from build123d import *

# Parameters (mm, degrees)
SKETCH1_R           = 5
BOSS_EXTRUDE1_DEPTH = 18
SKETCH2_R           = 2.27
CUT_EXTRUDE1_DEPTH  = 5.68
CUT_EXTRUDE1_TAPER  = 3.074
SKETCH7_R           = 1
CUT_EXTRUDE2_DEPTH  = 19
SKETCH9_R           = 2.27
CUT_EXTRUDE3_DEPTH  = 5.68
CUT_EXTRUDE3_TAPER  = 3.074


with BuildPart() as part:
    # Sketch1 → Boss-Extrude1 (new body)
    with BuildSketch(Plane.XY):
        Circle(SKETCH1_R)
    extrude(amount=BOSS_EXTRUDE1_DEPTH)

    # Sketch2 → Cut-Extrude1 (cut)
    with BuildSketch(Plane.XY):
        Circle(SKETCH2_R)
    extrude(amount=CUT_EXTRUDE1_DEPTH, taper=CUT_EXTRUDE1_TAPER, mode=Mode.SUBTRACT)

    # Sketch7 → Cut-Extrude2 (cut, through all)
    with BuildSketch(Plane.XY):
        Circle(SKETCH7_R)
    extrude(amount=CUT_EXTRUDE2_DEPTH, mode=Mode.SUBTRACT)

    # Sketch9 → Cut-Extrude3 (cut)
    with BuildSketch(Plane.XY.offset(18)):
        Circle(SKETCH9_R)
    extrude(amount=-CUT_EXTRUDE3_DEPTH, taper=CUT_EXTRUDE3_TAPER, mode=Mode.SUBTRACT)


solid = part.part
Here's how the part is built. I have some questions about the finished solid (model axes, mm). A direction names the side the tool comes from. Round coordinates to 2 decimals unless told otherwise and drop trailing zeros. Write each loop counter-clockwise with the first axis right and the second up, starting at its lowest first coordinate (ties: lowest second). Pieces come first, ordered by that corner, then holes.
1. Suppose I cut it at C-C (z = 16.25). List the corners of the cut face in (x, y) for me, and give its area (3 significant figures).
2. Suppose I cut it at D-D (z = 10.5). List the corners of the cut face in (x, y) for me.
3. I need wall thicknesses on L1, parallel to Y at x = 0, z = 9.5; L2, parallel to Y at x = -0.5, z = 1.75; L3, parallel to X at y = 1.5, z = 5. Which ranges of each line are inside material? Lowest first, please.
4. Will these pins go through, and if not, where does the flat tip stop? pin 1 Ø1 at (y, z) = (-3, 14.5) entering from -X; pin 2 Ø5 at (y, z) = (-1.5, 10) entering from -X; pin 3 Ø1 at (x, z) = (2.5, 5.5) entering from +Y; pin 4 Ø1.2 at (x, y) = (1, 0) entering from +Z.
5. Suppose I cut it at A-A (x = 0). List the corners of the cut face in (y, z) for me, and give its area (3 significant figures).
6. For faces 1 (the flat face through (1, -1, 12.32)), 2 (the conical face through (2.018, 0.635, 2.88)), which set-ups out of +Z, -Z, +X, -X, +Y, -Y let a thin tool reach every point of the face, with its end or its side?
7. If we mould it in two halves opening along Y, with no side actions, what happens to faces 3 (the flat face through (2.2, 1.2, 0)), 4 (the cylindrical face through (-1.08, -4.88, 8.87)), 5 (the flat face through (1, -1, 5.68))? For each: released by +Y, released by -Y, zero draft, split by the parting line, or undercut.
8. Suppose I cut it at B-B (y = 3). List the corners of the cut face in (x, z) for me, and give its area (3 significant figures).
Answer sheet:
1. outline: circle Ø10 at (0, 0); hole circle Ø4.35 at (0, 0)
1. area: 63.7 mm2
2. outline: circle Ø10 at (0, 0); hole circle Ø2 at (0, 0)
3. L1: y = -5 to -1, 1 to 5
3. L2: y = -4.97 to -2.12, 2.12 to 4.97
3. L3: x = -4.77 to -1.33, 1.33 to 4.77
4. pin 1: stops at x = -4.33
4. pin 2: stops at x = -5
4. pin 3: stops at y = 4.58
4. pin 4: stops at z = 12.32
5. outline: (-5, 0) - (-2.27, 0) - (-1.96, 5.68) - (-1, 5.68) - (-1, 12.32) - (-1.96, 12.32) - (-2.27, 18) - (-5, 18) - close; (1, 5.68) - (1.96, 5.68) - (2.27, 0) - (5, 0) - (5, 18) - (2.27, 18) - (1.96, 12.32) - (1, 12.32) - close
5. area: 119 mm2
6. face 1: +Z
6. face 2: -Z
7. face 3: zero draft
7. face 4: split by the parting line
7. face 5: undercut
8. outline: (-4, 0) - (4, 0) - (4, 18) - (-4, 18) - close
8. area: 144 mm2
